```python
from build123d import *

# Parameters (mm, degrees)
EXTRUDE_2_DEPTH          = 100
CUT_EXTRUDE_1_DEPTH      = 143.286557619
CUT_EXTRUDE_1_DEPTH_BACK = 143.286557619
EXTRUDE_3_DEPTH          = 10


with BuildPart() as part:
    # 草图5 → 拉伸-薄壁2 (new body)
    with BuildSketch(Plane(origin=(0, 0, 0), x_dir=(1, 0, 0), z_dir=(0, 1, 0))):
        Polygon((-85.11384198, 46.497376637), (0, 0), (83.416414932, 46.497376637), (88.285235684, 37.762699512), (0.048663646, -11.421494349), (-89.908055505, 37.72152815), align=None)
    extrude(amount=EXTRUDE_2_DEPTH)

    # 草图6 → 切除-拉伸1 (cut, two sides: drawn at the far end of the back side and taken through both)
    with BuildSketch(Plane(origin=(0, 0, 0), x_dir=(0, 0, -1), z_dir=(1, 0, 0)).offset(-CUT_EXTRUDE_1_DEPTH_BACK)):
        Polygon((-11.421494349, 0), (46.497376637, 26.437958822), (46.497376637, 0), align=None)
        Polygon((46.497376637, 100), (-11.421494349, 73.562041178), (-11.421494349, 100), align=None)
    extrude(amount=CUT_EXTRUDE_1_DEPTH + CUT_EXTRUDE_1_DEPTH_BACK, mode=Mode.SUBTRACT)

    # 草图7 → 凸台-拉伸3 (add)
    with BuildSketch(Plane(origin=(0, 65.192092202, 29.757932429), x_dir=(1, 0, 0), z_dir=(0, 0.909707375853676, 0.4152499130853836))):
        Polygon((88.285235684, 74.222363952), (83.416414932, 83.823997793), (58.456022425, 129.045976045), (-62.639885843, 129.045976045), (-85.11384198, 83.823997793), (-89.908055505, 74.177106144), (0.048663646, 20.156413552), align=None)
    extrude(amount=EXTRUDE_3_DEPTH)


solid = part.part
```
Work out the finished part from the listing and answer in its coordinate system (mm). A direction names the side the tool comes from. Round coordinates to 2 decimals unless told otherwise and drop trailing zeros. Loops run counter-clockwise (first coordinate to the right, second up) from the corner with the lowest first, then second, coordinate; pieces in that order, holes last.
(1) The part is cut by section B-B, the plane y = 54.5. Give the vertices of the cut face in (x, z).
Computed values:
outline: (-89.91, -37.72) - (-85.11, -46.5) - (0, 0) - (83.42, -46.5) - (88.29, -37.76) - (0.05, 11.42) - close
(2) The part is cut by section C-C, the plane z = -11.5. Give the vertices of the cut face in (x, y), and give its area (3 significant figures).
Computed values:
outline: (-49.51, 95.02) - (-41.91, 84.02) - (-41.91, 10.46) - (-21.05, 10.46) - (-21.05, 84.02) - (20.63, 84.02) - (20.63, 10.46) - (41.17, 10.46) - (41.17, 84.02) - (48.62, 95.02) - close
area: 4,040 mm2
(3) The mould has two halves that part along X. Classify faces 1 (the flat face through (-45.559, 89.42, -11.447)), 2 (the flat face through (85.817, 60.683, -42.191)), 3 (the flat face through (-43.2, 51.9, -23.6)), 4 (the flat face through (41.12, 51.94, -22.92)): pulls with the +X half, pulls with the -X half, needs draft (parallel to the pull), parting line crosses it, or undercut.
Computed values:
face 1: pulls with the -X half
face 2: pulls with the +X half
face 3: undercut
face 4: undercut
(4) The part is cut by section D-D, the plane x = -9.5. Give the vertices of the cut face in (y, z), and give its area (3 significant figures).
Computed values:
outline: (2.38, 6.21) - (7.58, -5.19) - (81.14, -5.19) - (118.78, -87.64) - (127.88, -83.48) - (85.04, 10.36) - (75.94, 6.21) - close
area: 1,870 mm2
(5) Each of these flat-tipped pins is pushed along its axis until it touches: P1, Ø1, axis at x = 50, y = 39.5, coming from the +Z side; P2, Ø3, axis at x = -33.5, z = -26.5, coming from the +Y side; P3, Ø6, axis at x = -19, y = 67, coming from the -Z side. Where does it stop, or does it pass through?
Computed values:
P1: stops at z = -16.14
P2: stops at y = 102.55
P3: stops at z = -12.02
(6) The part is cut by section A-A, the plane x = 26.5. Give the vertices of the cut face in (y, z).
Computed values:
outline: (6.73, -3.32) - (11.96, -14.77) - (85.52, -14.77) - (118.78, -87.64) - (127.88, -83.48) - (89.39, 0.83) - (80.29, -3.32) - close
(7) For faces 5 (the flat face through (-2.028, 103.502, -54.169)), 6 (the flat face through (44.785, 47.334, -13.515)), 7 (the flat face through (-1.24, 123.26, -85.59)), 8 (the flat face through (-44.3, 47.325, -12.806)), determine the directions among +Z, -Z, +X, -X, +Y, -Y from which every point of the face is accessible in a straight line to the end or side of a thin tool.
Computed values:
face 5: -Z, -Y
face 6: +Z, +X, -Y
face 7: -Z, +X, -X, +Y
face 8: +Z, -X, -Y
(8) Find the intervals of material crossed by L1, parallel to X at y = 49, z = -3; L2, parallel to X at y = 27, z = -15; L3, parallel to Z at x = 74, y = 57.5, in increasing order.
Computed values:
L1: x = -26.35 to -5.49, 5.38 to 25.92
L2: x = -48.32 to -27.46, 26.91 to 47.45
L3: z = -41.25 to -29.8
